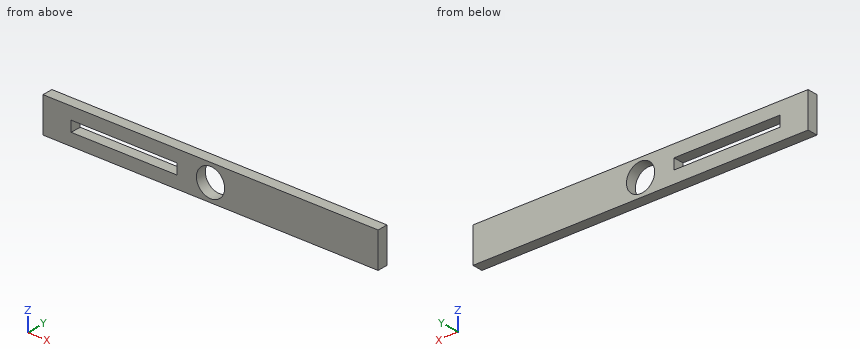
```python
from build123d import *

# Parameters (mm, degrees)
CROQUIS1_W              = 95
CROQUIS1_H              = 10
CROQUIS1_R              = 4
CROQUIS1_W_2            = 30
CROQUIS1_H_2            = 3
SALIENTE_EXTRUIR1_DEPTH = 3


with BuildPart() as part:
    # Croquis1 → Saliente-Extruir1 (new body)
    with BuildSketch(Plane(origin=(0, 0, 0), x_dir=(1, 0, 0), z_dir=(0, 1, 0))):
        Rectangle(CROQUIS1_W, CROQUIS1_H)
        Circle(CROQUIS1_R, mode=Mode.SUBTRACT)
        with Locations((-24.5, 0)):
            Rectangle(CROQUIS1_W_2, CROQUIS1_H_2, mode=Mode.SUBTRACT)
    extrude(amount=SALIENTE_EXTRUIR1_DEPTH)


solid = part.part
```
Work out the finished part from the listing and answer in its coordinate system (mm). Coordinates: 2 decimals unless noted, no trailing zeros. Order: outer loops, then holes, each group sorted by start corner. A loop starts at its lowest first (then second) coordinate and runs counter-clockwise, first axis right, second up. Notation, with made-up numbers: (-9.5, 7) - (48.5, 7) arc R21 cw to (48.5, 21) - close; hole circle Ø9 at (82, 2.25). An arc over 180 degrees is marked (long way). Answer as a JSON object with one key per item and string values.
1. Find section D-D on x = -37. Determine the outline of the cut face in (y, z), plus the area to 3 significant figures.
Output values:
{"outline": "(0, -5) - (3, -5) - (3, -1.5) - (0, -1.5) - close; (0, 1.5) - (3, 1.5) - (3, 5) - (0, 5) - close", "area": "21.0 mm²"}
2. Find section B-B on x = 0. Determine the outline of the cut face in (y, z).
Output values:
{"outline": "(0, -5) - (3, -5) - (3, -4) - (0, -4) - close; (0, 4) - (3, 4) - (3, 5) - (0, 5) - close"}
3. Consider line 1 (X direction, y = 1.9, z = 0); line 2 (Z direction, x = -36, y = 1.25); line 3 (Z direction, x = 0, y = 1.6). Determine where each line is inside the solid, lowest interval first.
Output values:
{"line 1": "x = -47.5 to -39.5, -9.5 to -4, 4 to 47.5", "line 2": "z = -5 to -1.5, 1.5 to 5", "line 3": "z = -5 to -4, 4 to 5"}
4. Find section C-C on z = 0. Determine the outline of the cut face in (x, y), plus the area to 3 significant figures.
Output values:
{"outline": "(-47.5, 0) - (-39.5, 0) - (-39.5, 3) - (-47.5, 3) - close; (-9.5, 0) - (-4, 0) - (-4, 3) - (-9.5, 3) - close; (4, 0) - (47.5, 0) - (47.5, 3) - (4, 3) - close", "area": "171 mm²"}
5. Find section A-A on y = 2.1. Determine the outline of the cut face in (x, z).
Output values:
{"outline": "(-47.5, -5) - (47.5, -5) - (47.5, 5) - (-47.5, 5) - close; hole (-39.5, -1.5) - (-9.5, -1.5) - (-9.5, 1.5) - (-39.5, 1.5) - close; hole circle Ø8 at (0, 0)"}
